Geometry check sheet. Reference: the model listing, model coordinates, mm. A direction names the side the tool comes from. Coordinates: 2 decimals unless noted, no trailing zeros. Loops run counter-clockwise (first coordinate to the right, second up) from the corner with the lowest first, then second, coordinate; pieces in that order, holes last. Notation, with made-up numbers: (12.5, 29) - (69.5, 29) arc R33 ccw to (69.5, 60) - close; hole circle Ø5 at (-20, 85.5). An arc over 180 degrees is marked (long way). Write each question's results on one line, items separated by ' | '. Start each with the question number.
(1) Sectioned sample at D-D (z = 38.5). Enter the section's corners in (x, y) (1 decimal).
(2) Mould release check, pull along X, two halves, no side actions. Record for faces 3 (the face through (0, 40, 15.773)), 4 (the face through (23.504, 30.824, 7.776)), 5 (the face through (-23.373, 31.556, 7.776)), 6 (the face through (-4.826, 16, 20)): pulls with the +X half, pulls with the -X half, needs draft (parallel to the pull), parting line crosses it, or undercut.
(3) Sectioned sample at B-B (x = 0). State how many separate pieces and enclosed holes the cut face has, plus the area to 3 significant figures.
(4) Go/stop test with flat-tipped pins: pin 1 Ø7.5 at (x, z) = (2, 19.5) entering from -Y (3 decimals); pin 2 Ø5.5 at (y, z) = (17, 19) entering from +X; pin 3 Ø1.5 at (y, z) = (9.5, 7.5) entering from +X. Record where each tip stops, or that it passes through.
(5) Access from +Z, -Z, +X, -X, +Y, -Y to the whole of each face (thin tool, end or side, straight path). Record for faces 1 (the face through (0.37, 73.02, 7.78)), 2 (the face through (0, 18.529, 20)).
(6) Material ranges on probe 1 along Y at (x, z) = (0, 9) (1 decimal); probe 2 along Y at (x, z) = (0, 16) (1 decimal); probe 3 along Y at (x, z) = (-4.5, 2.5), recorded low to high.
from build123d import *

# Parameters (mm, degrees)
F1_DEPTH = 40.2336
F2_R     = 3.302
F0_R     = 10.16
F3_DEPTH = 15.7734


with BuildPart() as f1:
    # F0 (on Top) → F1 (new body)
    with BuildSketch(Plane.XY):
        with BuildLine():
            ThreePointArc((-28.126541, 5.042647), (-2.531275, -28.462665), (28.575, 0))
            ThreePointArc((28.575, 0), (28.462665, 2.531275), (28.126541, 5.042647))
            ThreePointArc((28.126541, 5.042647), (0, 28.575), (-28.126541, 5.042647))
        make_face()
        with BuildLine():
            ThreePointArc((4.826, 13.447765), (11.685122, 8.22135), (14.2875, 0))
            ThreePointArc((14.2875, 0), (-8.22135, -11.685122), (-4.826, 13.447765))
            Line((-4.826, 13.447765), (-4.826, 18.5293))
            Line((-4.826, 18.5293), (0, 18.5293))
            Line((0, 18.5293), (4.826, 18.5293))
            Line((4.826, 18.5293), (4.826, 13.447765))
        make_face(mode=Mode.SUBTRACT)
    extrude(amount=F1_DEPTH)

    # F2
    f2_edges = [f1.edges().sort_by_distance(p)[0] for p in [
        (-28.575, 0, 40.2336),
    ]]
    fillet(f2_edges, radius=F2_R)

    # F0 (on Top) → F3 (join)
    with BuildSketch(Plane.XY):
        with BuildLine():
            ThreePointArc((-28.126541, 5.042647), (0, 28.575), (28.126541, 5.042647))
            Line((28.126541, 5.042647), (18.751028, 57.336765))
            ThreePointArc((18.751028, 57.336765), (18.97511, 55.662516), (19.05, 53.975))
            ThreePointArc((19.05, 53.975), (-1.687516, 34.99989), (-18.751028, 57.336765))
            Line((-18.751028, 57.336765), (-28.126541, 5.042647))
        make_face()
        with BuildLine():
            ThreePointArc((19.05, 53.975), (18.97511, 55.662516), (18.751028, 57.336765))
            ThreePointArc((18.751028, 57.336765), (0, 73.025), (-18.751028, 57.336765))
            ThreePointArc((-18.751028, 57.336765), (-1.687516, 34.99989), (19.05, 53.975))
        make_face()
        with Locations((0, 53.975)):
            Circle(F0_R, mode=Mode.SUBTRACT)
    extrude(amount=F3_DEPTH)


solid = f1.part
Outcome:
1) outline: (-27.7, 5) arc R28.2 ccw (long way) to (28.2, 0) arc R28.2 ccw to (27.7, 5) arc R28.2 ccw to start; hole (-4.8, 13.4) arc R14.3 ccw (long way) to (14.3, 0) arc R14.3 ccw to (4.8, 13.4) - (4.8, 18.5) - (-4.8, 18.5) - close
2) face 3: needs draft | face 4: pulls with the +X half | face 5: pulls with the -X half | face 6: undercut
3) separate pieces: 3 | enclosed holes: 0 | area: 1,350 mm2
4) pin 1: stops at y = -28.575 | pin 2: stops at x = 24.77 | pin 3: stops at x = 27.46
5) face 1: +Z, -Z, +Y | face 2: +Z, -Z
6) probe 1: y = -28.6 to -14.3, 18.5 to 43.8, 64.1 to 73 | probe 2: y = -28.6 to -14.3, 18.5 to 28.6 | probe 3: y = -28.22 to -13.56, 18.53 to 44.87, 63.08 to 72.49
